Geometry: final body of the model. Coordinates: model frame, mm. A direction names the side the tool comes from. Give positions to 0.01 mm unless a question says otherwise; leave off trailing zeros. Loops run counter-clockwise (first coordinate to the right, second up) from the corner with the lowest first, then second, coordinate; pieces in that order, holes last. Notation, with made-up numbers: M -37.5,64 L -8.5,64 A18 ccw -8.5,77 Z; hole C -26,-17 d4. An arc over 180 degrees is marked long. Put each result on its own line as item: value.
```python
from build123d import *

# Parameters (mm, degrees)
F0_W      = 35
F0_H      = 30
F1_DEPTH  = 150
F2_W      = 28
F2_H      = 21
F3_DEPTH  = 48
F4_W      = 22
F4_H      = 15
F5_DEPTH  = 85.9
F6_R      = 6.5
F7_DEPTH  = 15
F9_W      = 5.382292
F9_H      = 69.969817
F10_DEPTH = 5
F11_R     = 7.5
F12_DEPTH = 133


with BuildPart() as f1:
    # F0 (on Top) → F1 (new body)
    with BuildSketch(Plane.XY):
        Rectangle(F0_W, F0_H)
    extrude(amount=F1_DEPTH)

    # F2 (on face) → F3 (cut)
    with BuildSketch(Plane.XY.offset(150)):
        Rectangle(F2_W, F2_H)
    extrude(amount=-F3_DEPTH, mode=Mode.SUBTRACT)

    # F4 (on face) → F5 (cut)
    with BuildSketch(Plane.XY.offset(150)):
        Rectangle(F4_W, F4_H)
    extrude(amount=-F5_DEPTH, mode=Mode.SUBTRACT)

    # F6 (on face) → F7 (cut)
    with BuildSketch(Plane.YZ.offset(17.5)):
        with Locations((0, 26.118774)):
            Circle(F6_R)
    extrude(amount=-F7_DEPTH, mode=Mode.SUBTRACT)

    # F9 (on face) → F10 (cut)
    with BuildSketch(Plane.YZ.offset(17.5)):
        with Locations((0, 150.352105)):
            Rectangle(F9_W, F9_H)
    extrude(amount=-F10_DEPTH, mode=Mode.SUBTRACT)

    # F11 (on face) → F12 (cut)
    with BuildSketch(Plane.XY.offset(150)):
        Circle(F11_R)
    extrude(amount=-F12_DEPTH, mode=Mode.SUBTRACT)


solid = f1.part
```
Item 1: Section C-C on z = 131. Output: boundary loops of the cut face in (x, y), then the cut area to 3 significant figures.
Output values:
outline: M -17.5,-15 L 17.5,-15 L 17.5,-2.69 L 14,-2.69 L 14,-10.5 L -14,-10.5 L -14,10.5 L 14,10.5 L 14,2.69 L 17.5,2.69 L 17.5,15 L -17.5,15 Z
area: 443 mm²
Item 2: Mould query, pull axis Z, two halves, no side actions, for faces 4 (the flat face through (0, -9, 102)), 5 (the flat face through (14, -5, 126)), 6 (the flat face through (0, 0, 0)), 7 (the cylindrical face through (12.246, 6.004, 23.629)). Classes: pulls with the +Z half, pulls with the -Z half, needs draft (parallel to the pull), parting line crosses it, or undercut.
Output values:
face 4: pulls with the +Z half
face 5: needs draft
face 6: pulls with the -Z half
face 7: undercut
Item 3: Section D-D on x = -5.5. Output: boundary loops of the cut face in (y, z), then the cut area to 3 significant figures.
Output values:
outline: M -15,0 L 15,0 L 15,150 L 10.5,150 L 10.5,102 L 7.5,102 L 7.5,64.1 L 5.1,64.1 L 5.1,17 L -5.1,17 L -5.1,64.1 L -7.5,64.1 L -7.5,102 L -10.5,102 L -10.5,150 L -15,150 Z
area: 2,440 mm²
Item 4: Pin query (flat end, axial travel): pin 1 Ø2 at (x, y) = (-3.5, 3) entering from +Z; pin 2 Ø5.5 at (x, y) = (5, 3) entering from +Z; pin 3 Ø8 at (x, y) = (2.5, -4.5) entering from +Z. Return the tip coordinate at first contact, or that it passes through.
Output values:
pin 1: z = 17
pin 2: z = 64.1
pin 3: z = 102
Item 5: Line query: probe 1 along Z at (x, y) = (12.5, 0); probe 2 along X at (y, z) = (6.75, 69.5); probe 3 along X at (y, z) = (0, 41). Output: solid intervals per line, ascending. Write a range as [from, to].
Output values:
probe 1: [0, 19.62], [32.62, 102]
probe 2: [-17.5, -11], [11, 17.5]
probe 3: [-17.5, -7.5], [7.5, 17.5]
Item 6: Section A-A on z = 106. Output: boundary loops of the cut face in (x, y).
Output values:
outline: M -17.5,-15 L 17.5,-15 L 17.5,15 L -17.5,15 Z; hole M -14,-10.5 L 14,-10.5 L 14,10.5 L -14,10.5 Z
Item 7: Set-up query: faces 1 (the flat face through (0, -15, 74)), 2 (the flat face through (16, -2.691, 132)), 3 (the flat face through (-14, 0, 126)). Return all of +Z, -Z, +X, -X, +Y, -Y with unobstructed straight access to the full face (end or side cutting, diameter ignored); none if empty.
Output values:
face 1: +Z, -Z, +X, -X, -Y
face 2: +Z, +X
face 3: +Z
Item 8: Section B-B on y = 0. Output: boundary loops of the cut face in (x, z).
Output values:
outline: M -17.5,0 L 17.5,0 L 17.5,19.62 L 7.5,19.62 L 7.5,17 L -7.5,17 L -7.5,64.1 L -11,64.1 L -11,102 L -14,102 L -14,150 L -17.5,150 Z; M 7.5,32.62 L 17.5,32.62 L 17.5,115.37 L 14,115.37 L 14,102 L 11,102 L 11,64.1 L 7.5,64.1 Z
